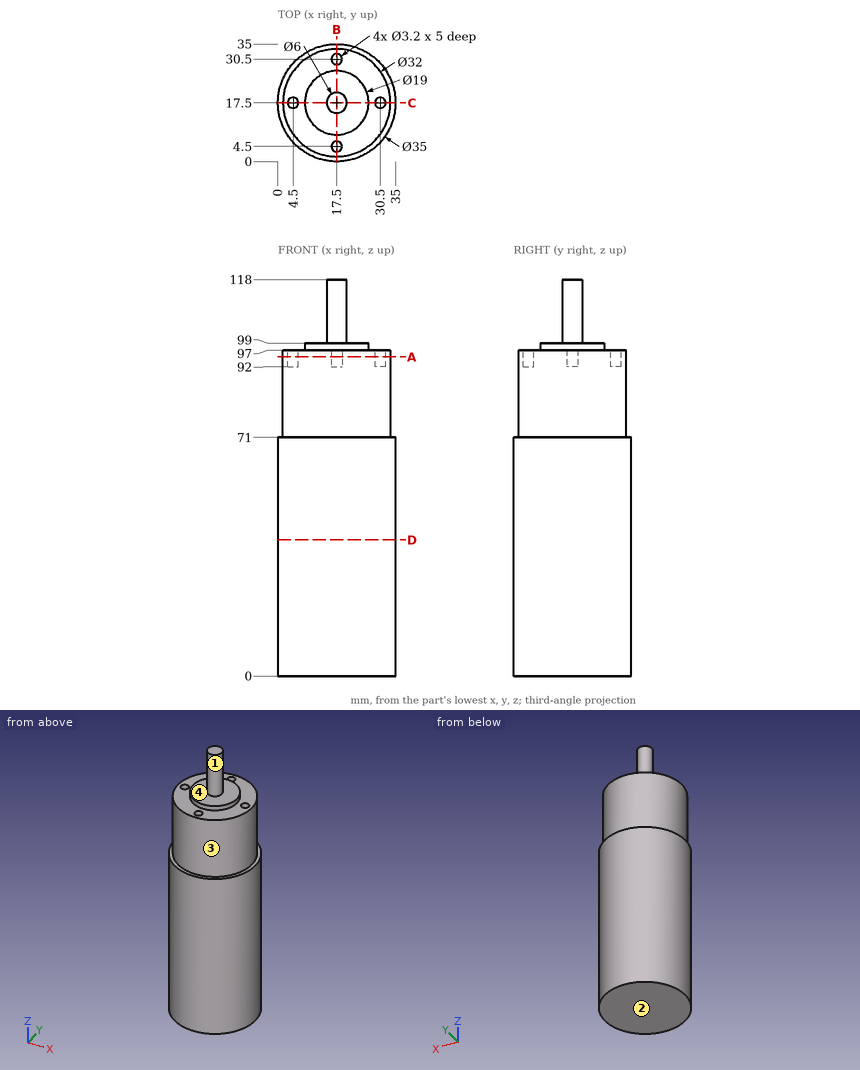
Can you work these out from the drawing? Everything is in mm from the part's minimum corner. A direction names the side the tool comes from. Round coordinates to 2 decimals unless told otherwise and drop trailing zeros. Loops run counter-clockwise (first coordinate to the right, second up) from the corner with the lowest first, then second, coordinate; pieces in that order, holes last. Notation, with made-up numbers: (-38, 56) - (-14, 56) arc R31 cw to (-14, 93) - close; hole circle Ø6 at (-35.5, 58.25). An arc over 180 degrees is marked (long way). Answer in a Markdown table with one row per item. Add a question column.
(1) I need wall thicknesses on line 1 along Y through (x, z) = (17.5, 95.3); line 2 along Y through (x, z) = (17, 93); line 3 along Z through (x, y) = (16.5, 14). Which ranges of each line are inside material? Lowest first, please.
(2) If we section it at A-A (z = 95): Please give me the cut outline in (x, y).
(3) If we mould it in two halves opening along X, with no side actions, what happens to the marked faces 3 and 4? For each: pulls with the +X half, pulls with the -X half, needs draft (parallel to the pull), parting line crosses it, or undercut.
(4) I'm going to push flat-ended pins straight in: pin 1 (6 mm diameter, centred on x = 17, z = 105.5, fed in from -Y); pin 2 (10.5 mm diameter, centred on x = 16.5, y = 22.5, fed in from +Z); pin 3 (4 mm diameter, centred on x = 14.5, z = 88, fed in from +Y); pin 4 (4 mm diameter, centred on x = 17.5, y = 30.5, fed in from +Z). Where does each tip first touch, or does it pass through?
(5) If we section it at B-B (x = 17.5): Please give me the cut outline in (y, z).
(6) For the marked faces 1 and 2, which set-ups out of +Z, -Z, +X, -X, +Y, -Y let a thin tool reach every point of the face, with its end or its side?
(7) If we section it at D-D (z = 40.5): Please give me the cut outline in (x, y).
Model answer:
| question | item | result |
|---|---|---|
| 1 | line 1 | y = 1.5 to 2.9, 6.1 to 28.9, 32.1 to 33.5 |
| 1 | line 2 | y = 1.51 to 2.98, 6.02 to 28.98, 32.02 to 33.49 |
| 1 | line 3 | z = 0 to 99 |
| 2 | outline | circle Ø32 at (17.5, 17.5); hole circle Ø3.2 at (4.5, 17.5); hole circle Ø3.2 at (17.5, 4.5); hole circle Ø3.2 at (17.5, 30.5); hole circle Ø3.2 at (30.5, 17.5) |
| 3 | face 3 | parting line crosses it |
| 3 | face 4 | needs draft |
| 4 | pin 1 | stops at y = 14.5 |
| 4 | pin 2 | stops at z = 118 |
| 4 | pin 3 | stops at y = 33.47 |
| 4 | pin 4 | stops at z = 97 |
| 5 | outline | (0, 0) - (35, 0) - (35, 71) - (33.5, 71) - (33.5, 97) - (32.1, 97) - (32.1, 92) - (28.9, 92) - (28.9, 97) - (27, 97) - (27, 99) - (20.5, 99) - (20.5, 118) - (14.5, 118) - (14.5, 99) - (8, 99) - (8, 97) - (6.1, 97) - (6.1, 92) - (2.9, 92) - (2.9, 97) - (1.5, 97) - (1.5, 71) - (0, 71) - close |
| 6 | face 1 | +Z |
| 6 | face 2 | -Z, +X, -X, +Y, -Y |
| 7 | outline | circle Ø35 at (17.5, 17.5) |
